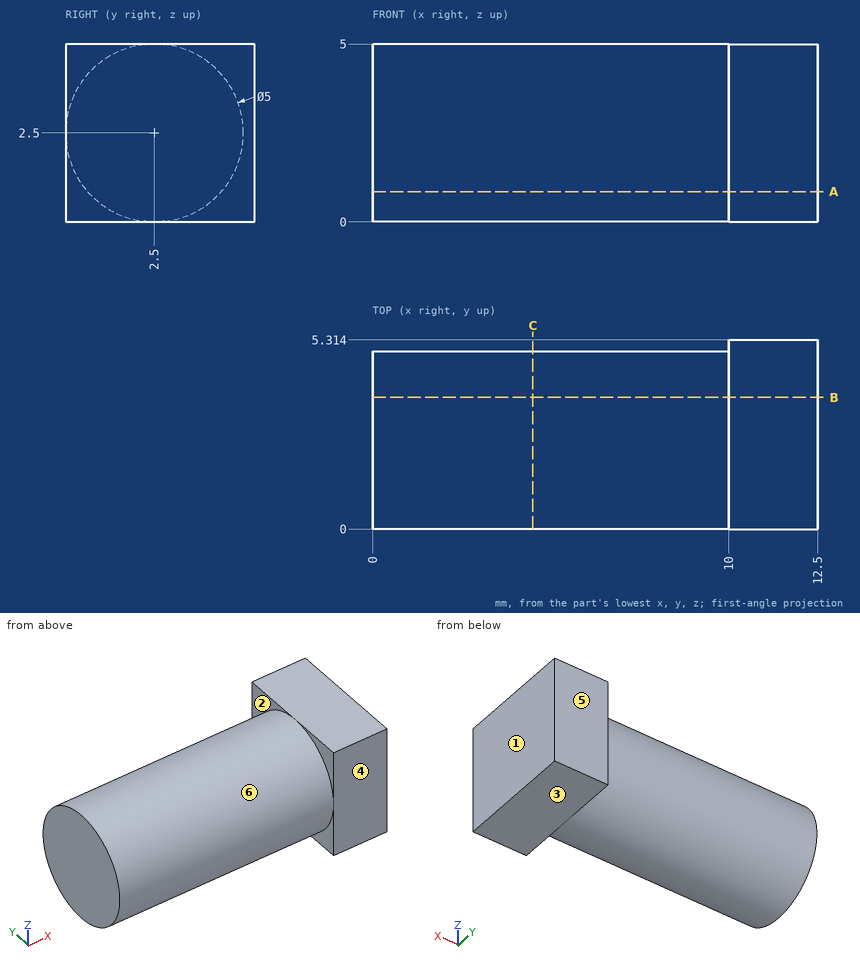
Check sheet for the drawn part. Datum: minimum x, y, z corner. Units: mm. A direction names the side the tool comes from. Coordinates: 2 decimals unless noted, no trailing zeros. Write each loop counter-clockwise with the first axis right and the second up, starting at its lowest first coordinate (ties: lowest second). Pieces come first, ordered by that corner, then holes. Notation, with made-up numbers: M -2.5,76 L 40.5,76 A17 cw 40.5,101 Z; hole C 61.25,89.5 d6. An arc over 180 degrees is marked long. One line per item, written item: value.
Item 1: Section check B-B, the plane y = 3.7. Record the boundary of the cut face in (x, z).
Check sheet entries:
outline: M 0,0.31 L 10,0.31 L 10,0 L 12.5,0 L 12.5,5 L 10,5 L 10,4.69 L 0,4.69 Z
Item 2: Gauge pin test, flat end, axial feed: pin 1 Ø1 at (x, z) = (2.5, 3.5) entering from +Y. Record the tip position at first contact, or that the pin passes through.
Check sheet entries:
pin 1: stops at y = 4.95
Item 3: Section check A-A, the plane z = 0.85. Record the boundary of the cut face in (x, y) (1 decimal).
Check sheet entries:
outline: M 0,0.6 L 10,0.6 L 10,0 L 12.5,0 L 12.5,5.3 L 10,5.3 L 10,4.4 L 0,4.4 Z
Item 4: Mould release check, pull along Y, two halves, no side actions. Record for the marked faces 3, 4, 5 and 6: pulls with the +Y half, pulls with the -Y half, needs draft (parallel to the pull), parting line crosses it, or undercut.
Check sheet entries:
face 3: needs draft
face 4: pulls with the -Y half
face 5: pulls with the +Y half
face 6: parting line crosses it
Item 5: Section check C-C, the plane x = 4.5. Record the boundary of the cut face in (y, z), plus the area to 3 significant figures.
Check sheet entries:
outline: C 2.5,2.5 d5
area: 19.6 mm^2
Item 6: Scan lines: line 1 along X through (y, z) = (4.9, 1.15); line 2 along Y through (x, z) = (9.25, 2.4); line 3 along Z through (x, y) = (3.25, 4). Record each from-to range of solid material in increasing order.
Check sheet entries:
line 1: x = 10 to 12.5
line 2: y = 0 to 5
line 3: z = 0.5 to 4.5
Item 7: Access from +Z, -Z, +X, -X, +Y, -Y to the whole of each face (thin tool, end or side, straight path). Record for the marked faces 1 and 2.
Check sheet entries:
face 1: +Z, -Z, +X, +Y, -Y
face 2: -X, +Y
